```python
from build123d import *

# Parameters (mm, degrees)
SKETCH2_R                = 100
BOSS_EXTRUDE1_DEPTH      = 120
SKETCH3_R                = 160
BOSS_EXTRUDE2_DEPTH      = 16
SKETCH5_R                = 130
SKETCH5_R_2              = 75
BOSS_EXTRUDE3_DEPTH      = 90
BOSS_EXTRUDE4_REACH      = 401.794
BOSS_EXTRUDE4_END_RADIUS = 130
SKETCH6_W                = 220
SKETCH6_H                = 160
FILLET1_R                = 10


with BuildPart() as part:
    # Sketch2 → Boss-Extrude1 (new body)
    with BuildSketch(Plane(origin=(0, 0, 0), x_dir=(1, 0, 0), z_dir=(0, 1, 0))):
        with Locations(Location((0.261683243, 0.036180985, 0), (0, 0, 270))):
            Circle(SKETCH2_R)
    extrude(amount=BOSS_EXTRUDE1_DEPTH)

    # Sketch3 → Boss-Extrude2 (add)
    with BuildSketch(Plane(origin=(0, 120, 0), x_dir=(1, 0, 0), z_dir=(0, 1, 0))):
        with Locations(Location((0.527861333, -0.229997105, 0), (0, 0, 270))):
            Circle(SKETCH3_R)
    extrude(amount=BOSS_EXTRUDE2_DEPTH)



with BuildPart() as body_2:
    # Sketch5 → Boss-Extrude3 (new, symmetric)
    with BuildSketch(Plane.XY):
        with Locations(Location((-7.162571242, 335.229832199, 0), (0, 0, 180))):
            Circle(SKETCH5_R)
        with Locations(Location((-8.194202002, 336, 0), (0, 0, 180))):
            Circle(SKETCH5_R_2, mode=Mode.SUBTRACT)
    extrude(amount=BOSS_EXTRUDE3_DEPTH, both=True)


with BuildPart() as part_1:
    add(part.part)

    add(body_2.part)  # Boss-Extrude4 merges body 2
    # Boss-Extrude4: up to this cylinder (the profile starts outside it)
    boss_extrude4_end = Plane(origin=(-7.162571242, 335.229832199, -0.621773), z_dir=(0, 0, -1)) * Cylinder(BOSS_EXTRUDE4_END_RADIUS, 1064.588, mode=Mode.PRIVATE)
    # Sketch6 → Boss-Extrude4 (add, up to the surface)
    with BuildSketch(Plane(origin=(0, 136, 0), x_dir=(1, 0, 0), z_dir=(0, 1, 0)), mode=Mode.PRIVATE) as boss_extrude4_sk1:
        with Locations((-9.267492371, 0.621772782)):
            Rectangle(SKETCH6_W, SKETCH6_H)
    boss_extrude4_tool1 = extrude(boss_extrude4_sk1.sketch, amount=BOSS_EXTRUDE4_REACH, mode=Mode.PRIVATE) - boss_extrude4_end
    add(boss_extrude4_tool1.solids().sort_by_distance((-9.267492, 136, -0.621773))[0])

    # Fillet1
    fillet1_edges = [part_1.edges().sort_by_distance(p)[0] for p in [
        (-119.267492371, 202.704102304, 79.378227218),
        (-119.267492371, 202.704102304, -80.621772782),
        (100.732507629, 199.356634441, 79.378227218),
        (100.732507629, 199.356634441, -80.621772782),
    ]]
    fillet(fillet1_edges, radius=FILLET1_R)


solid = part_1.part
```
Geometry: final body of the model. Coordinates: model frame, mm. A direction names the side the tool comes from. Round coordinates to 2 decimals unless told otherwise and drop trailing zeros. Write each loop counter-clockwise with the first axis right and the second up, starting at its lowest first coordinate (ties: lowest second). Pieces come first, ordered by that corner, then holes. Notation, with made-up numbers: M 6,-11.75 L 65,-11.75 A11 ccw 65,-5.75 Z; hole C -24,83 d11. An arc over 180 degrees is marked long. Answer in a Markdown table with one row per item. Add a question column.
(1) Draft query along Y for faces 1 (the face through (48.59, 127.89, 152.84)), 2 (the face through (97.88, 200.24, 76.37)), 3 (the face through (2, 0, -1)). Return one class per face: pulls with the +Y half, pulls with the -Y half, needs draft (parallel to the pull), parting line crosses it, or undercut.
(2) Reachability of faces 4 (the face through (-119.267, 202, 0)), 5 (the face through (-60.59, 59.16, -79.39)), 6 (the face through (-116.416, 203.638, 76.371)) from +Z, -Z, +X, -X, +Y, -Y: full face, straight path, thin tool, end or side. Return the list, or none.
(3) Ray query, L1, parallel to X at y = 336, z = -8; L2, parallel to Y at x = -63, z = 89; L3, parallel to Y at x = 0, z = -121. Return the intervals inside material, ascending.
(4) Cut plane A-A, the plane x = 26. Return the cut outline in (y, z), then the cut area to 3 significant figures.
(5) Cut plane C-C, the plane x = -32.5. Return the cut outline in (y, z), then the cut area to 3 significant figures.
(6) Contact query for flat-ended pins moving along their axis: pin 1 (1 mm diameter, centred on x = -77, y = 409.5, fed in from +Z); pin 2 (8 mm diameter, centred on x = -103.5, z = -47.5, fed in from -Y); pin 3 (10 mm diameter, centred on y = 164.5, z = -45, fed in from -X). Output: stop coordinate, or through.
(7) Cut plane D-D, the plane x = -91. Return the cut outline in (y, z).
(8) Cut plane B-B, the plane z = -42.5. Return the cut outline in (x, y), then the cut area to 3 significant figures.
Established:
| question | item | result |
|---|---|---|
| 1 | face 1 | needs draft |
| 1 | face 2 | undercut |
| 1 | face 3 | pulls with the -Y half |
| 2 | face 4 | +Z, -Z, -X |
| 2 | face 5 | -Y |
| 2 | face 6 | +Z, -X |
| 3 | L1 | -137.16 to -83.19, 66.81 to 122.84 |
| 3 | L2 | 120 to 136, 217.83 to 284.8, 387.2 to 452.63 |
| 3 | L3 | 120 to 136 |
| 4 | outline | M 0,-96.67 L 120,-96.67 L 120,-157.73 L 136,-157.73 L 136,-80.62 L 209.53,-80.62 L 209.53,-90 L 269.25,-90 L 269.25,90 L 209.53,90 L 209.53,79.38 L 136,79.38 L 136,158.19 L 120,158.19 L 120,96.59 L 0,96.59 Z; M 402.75,-90 L 460.93,-90 L 460.93,90 L 402.75,90 Z |
| 4 | area | 61,200 mm² |
| 5 | outline | M 0,-94.52 L 120,-94.52 L 120,-156.32 L 136,-156.32 L 136,-80.62 L 207.72,-80.62 L 207.72,-90 L 265.05,-90 L 265.05,90 L 207.72,90 L 207.72,79.38 L 136,79.38 L 136,156.78 L 120,156.78 L 120,94.44 L 0,94.44 Z; M 406.95,-90 L 462.74,-90 L 462.74,90 L 406.95,90 Z |
| 5 | area | 59,500 mm² |
| 6 | pin 1 | z = 90 |
| 6 | pin 2 | y = 120 |
| 6 | pin 3 | x = -119.27 |
| 7 | outline | M 0,-40.92 L 120,-40.92 L 120,-131.01 L 136,-131.01 L 136,-80.62 L 235.88,-80.62 L 235.88,-90 L 434.58,-90 L 434.58,90 L 235.88,90 L 235.88,79.38 L 136,79.38 L 136,131.47 L 120,131.47 L 120,40.85 L 0,40.85 Z |
| 8 | outline | M -153.66,120 L -90.27,120 L -90.27,0 L 90.8,0 L 90.8,120 L 154.72,120 L 154.72,136 L 100.73,136 L 100.73,262.71 A130 ccw long -119.27,269.41 L -119.27,136 L -153.66,136 Z; hole C -8.19,336 d150 |
| 8 | area | 81,300 mm² |
